from build123d import *

# Parameters (mm, degrees)
SKETCH1_R           = 1.35
SKETCH1_W           = 11
SKETCH1_H           = 69
BOSS_EXTRUDE1_DEPTH = 6.35
FILLET1_R           = 2


with BuildPart() as part:
    # Sketch1 → Boss-Extrude1 (new body)
    with BuildSketch(Plane(origin=(0, 0, 0), x_dir=(1, 0, 0), z_dir=(0, 1, 0))):
        with BuildLine():
            ThreePointArc((32.995567884, -67.352004425), (0, 75), (-32.995567884, -67.352004425))
            ThreePointArc((-32.995567884, -67.352004425), (0, -48.302004425), (32.995567884, -67.352004425))
        make_face()
        with Locations((-42.910067426, 18.208347884)):
            Circle(SKETCH1_R, mode=Mode.SUBTRACT)
        with Locations((42.910067426, 18.208347884)):
            Circle(SKETCH1_R, mode=Mode.SUBTRACT)
        with Locations((-33.21799214, 49)):
            Circle(SKETCH1_R, mode=Mode.SUBTRACT)
        with Locations((-4.78200786, 49)):
            Circle(SKETCH1_R, mode=Mode.SUBTRACT)
        with Locations((4.78200786, 49)):
            Circle(SKETCH1_R, mode=Mode.SUBTRACT)
        with Locations((33.21799214, 49)):
            Circle(SKETCH1_R, mode=Mode.SUBTRACT)
        with Locations((-42.910067426, 11.1)):
            Circle(SKETCH1_R, mode=Mode.SUBTRACT)
        with Locations((-42.910067426, -11.1)):
            Circle(SKETCH1_R, mode=Mode.SUBTRACT)
        with Locations((-11.160067426, -11.1)):
            Circle(SKETCH1_R, mode=Mode.SUBTRACT)
        with Locations((-11.160067426, 11.1)):
            Circle(SKETCH1_R, mode=Mode.SUBTRACT)
        with Locations((11.160067426, 11.1)):
            Circle(SKETCH1_R, mode=Mode.SUBTRACT)
        with Locations((11.160067426, -11.1)):
            Circle(SKETCH1_R, mode=Mode.SUBTRACT)
        with Locations((42.910067426, -11.1)):
            Circle(SKETCH1_R, mode=Mode.SUBTRACT)
        with Locations((42.910067426, 11.1)):
            Circle(SKETCH1_R, mode=Mode.SUBTRACT)
        with Locations((45.192446616, 32.037646433)):
            Circle(SKETCH1_R, mode=Mode.SUBTRACT)
        with Locations((-45.192446616, 32.037646433)):
            Circle(SKETCH1_R, mode=Mode.SUBTRACT)
        with Locations((13.346873881, 34.693819966)):
            Circle(SKETCH1_R, mode=Mode.SUBTRACT)
        with Locations((-6.55476095, -38.026099982)):
            Circle(SKETCH1_R, mode=Mode.SUBTRACT)
        with Locations((-13.346873881, 34.693819966)):
            Circle(SKETCH1_R, mode=Mode.SUBTRACT)
        with Locations((10.597026674, -15.930038136)):
            Circle(SKETCH1_R, mode=Mode.SUBTRACT)
        with Locations((-38.234289702, -39.23697625)):
            Circle(SKETCH1_R, mode=Mode.SUBTRACT)
        with Locations((-43.68503018, -41.129285651)):
            Circle(SKETCH1_R, mode=Mode.SUBTRACT)
        with Locations((-43.68503018, 41.129285651)):
            Circle(SKETCH1_R, mode=Mode.SUBTRACT)
        with Locations((43.68503018, -41.129285651)):
            Circle(SKETCH1_R, mode=Mode.SUBTRACT)
        with Locations((43.68503018, 41.129285651)):
            Circle(SKETCH1_R, mode=Mode.SUBTRACT)
        with Locations((-44.385223141, -22.074211772)):
            Circle(SKETCH1_R, mode=Mode.SUBTRACT)
        with Locations((41.601681906, -17.457756634)):
            Circle(SKETCH1_R, mode=Mode.SUBTRACT)
        with Locations((38.234289702, -39.23697625)):
            Circle(SKETCH1_R, mode=Mode.SUBTRACT)
        with Locations((58.910067426, 0.102907352)):
            Rectangle(SKETCH1_W, SKETCH1_H, mode=Mode.SUBTRACT)
        with Locations((-58.910067426, 0.102907352)):
            Rectangle(SKETCH1_W, SKETCH1_H, mode=Mode.SUBTRACT)
        with BuildLine():
            ThreePointArc((-5.853899988, 64.744946271), (0.003726822, 68.153564176), (5.857575472, 64.738461857))
            ThreePointArc((5.857575472, 64.738461857), (10.16, 61.422565207), (5.857575472, 58.106668557))
            ThreePointArc((5.857575472, 58.106668557), (0.003726822, 54.691566239), (-5.853899988, 58.100184144))
            ThreePointArc((-5.853899988, 58.100184144), (-10.167207264, 61.422565207), (-5.853899988, 64.744946271))
        make_face(mode=Mode.SUBTRACT)
    extrude(amount=BOSS_EXTRUDE1_DEPTH)

    # Fillet1
    fillet1_edges = [part.edges().sort_by_distance(p)[0] for p in [
        (-32.995567884, 3.175, 67.352004425),
        (32.995567884, 3.175, 67.352004425),
    ]]
    fillet(fillet1_edges, radius=FILLET1_R)


solid = part.part
Work out the finished part from the listing and answer in its coordinate system (mm). A direction names the side the tool comes from. Coordinates: 2 decimals unless noted, no trailing zeros. Loops run counter-clockwise (first coordinate to the right, second up) from the corner with the lowest first, then second, coordinate; pieces in that order, holes last. Notation, with made-up numbers: (77, 69) -> (131, 69) arc R7 ccw to (131, 77) -> close; hole circle Ø9 at (54.5, 32). An arc over 180 degrees is marked (long way). Write each question's results on one line, items separated by ' | '. Start each with the question number.
1) Find section C-C on z = 52.5. Determine the outline of the cut face in (x, y).
2) Find section B-B on x = 0. Determine the outline of the cut face in (y, z), then the cut area to 3 significant figures.
3) Find section D-D on y = 5. Count the separate pieces of the cut face and the enclosed holes in it, then the cut area to 3 significant figures.
4) Find section A-A on z = 0. Determine the outline of the cut face in (x, y).
5) The mould has two halves that part along Z. Classify faces 1 (the flat face through (-1, 0, -5)), 2 (the cylindrical face through (-0.533, 3.131, 48.306)), 3 (the flat face through (-59, 3, 34.397)): pulls with the +Z half, pulls with the -Z half, needs draft (parallel to the pull), parting line crosses it, or undercut.
6) For faces 4 (the flat face through (-1, 6.35, -5)), 5 (the flat face through (-64.41, 3, 0)), determine the directions among +Z, -Z, +X, -X, +Y, -Y from which every point of the face is accessible in a straight line to the end or side of a thin tool.
7) Consider line 1 along X through (y, z) = (3.25, -32); line 2 along X through (y, z) = (4, 2.5); line 3 along X through (y, z) = (3.5, -27). Determine where each line is inside the solid, lowest interval first.
8) Flat-ended cylindrical pins translate along their axes: P1, Ø2, axis at x = 38.23, z = 39.24, coming from the +Y side; P2, Ø2, axis at x = -8.5, y = 5, coming from the -Z side; P3, Ø1, axis at x = 29.5, y = 4, coming from the -Z side; P4, Ø1.5, axis at x = -23.5, y = 4, coming from the +Z side. Find the tip coordinate at first contact, or state that the pin passes through.
Response values:
1) outline: (-53.56, 0) -> (-17.39, 0) -> (-17.39, 6.35) -> (-53.56, 6.35) -> close; (17.39, 0) -> (53.56, 0) -> (53.56, 6.35) -> (17.39, 6.35) -> close
2) outline: (0, -75) -> (6.35, -75) -> (6.35, -68.15) -> (0, -68.15) -> close; (0, -54.69) -> (6.35, -54.69) -> (6.35, 48.3) -> (0, 48.3) -> close | area: 697 mm^2
3) separate pieces: 1 | enclosed holes: 31 | area: 14,600 mm^2
4) outline: (-75, 0) -> (-64.41, 0) -> (-64.41, 6.35) -> (-75, 6.35) -> close; (-53.41, 0) -> (53.41, 0) -> (53.41, 6.35) -> (-53.41, 6.35) -> close; (64.41, 0) -> (75, 0) -> (75, 6.35) -> (64.41, 6.35) -> close
5) face 1: needs draft | face 2: pulls with the +Z half | face 3: undercut
6) face 4: +Z, -Z, +X, -X, +Y | face 5: +Y, -Y
7) line 1: x = -67.83 to -64.41, -53.41 to -46.54, -43.84 to 43.84, 46.54 to 53.41, 64.41 to 67.83 | line 2: x = -74.96 to -64.41, -53.41 to 53.41, 64.41 to 74.96 | line 3: x = -69.97 to -64.41, -53.41 to 53.41, 64.41 to 69.97
8) P1: passes through | P2: stops at z = -74.62 | P3: stops at z = -69.17 | P4: stops at z = 57.02
